```python
from build123d import *

# Parameters (mm, degrees)
F0_W     = 63.5
F0_H     = 5
F1_DEPTH = 10.5
F2_W     = 63.5
F2_H     = 25
F2_H_2   = 5
F3_DEPTH = 5
F4_SIZE  = 4.99999
F5_W     = 63.5
F5_H     = 5
F5_H_2   = 25
F6_DEPTH = 5
F7_SIZE  = 4.99999


# Not quite as in the source:
# - a fillet or chamfer is up to 0.001 mm smaller than in the source, because OpenCascade refuses the exact size


with BuildPart() as f1:
    # F0 (on Top) → F1 (new body)
    with BuildSketch(Plane.XY):
        Rectangle(F0_W, F0_H)
    extrude(amount=F1_DEPTH)

    # F2 (on face) → F3 (join)
    with BuildSketch(Plane.XY.offset(10.5)):
        with Locations((0, -15)):
            Rectangle(F2_W, F2_H)
        Rectangle(F2_W, F2_H_2)
    extrude(amount=F3_DEPTH)

    # F4 (size 5 in the source; OpenCascade refuses exactly that, so slightly less here)
    f4_edges = [f1.edges().sort_by_distance(p)[0] for p in [
        (0, -27.5, 15.5),
    ]]
    chamfer(f4_edges, length=F4_SIZE)

    # F5 (on face) → F6 (join)
    with BuildSketch(Plane(origin=(0, 0, 0), x_dir=(1, 0, 0), z_dir=(0, 0, -1))):
        Rectangle(F5_W, F5_H)
        with Locations((0, 15)):
            Rectangle(F5_W, F5_H_2)
    extrude(amount=F6_DEPTH)

    # F7 (size 5 in the source; OpenCascade refuses exactly that, so slightly less here)
    f7_edges = [f1.edges().sort_by_distance(p)[0] for p in [
        (0, -27.5, -5),
    ]]
    chamfer(f7_edges, length=F7_SIZE)


solid = f1.part
```
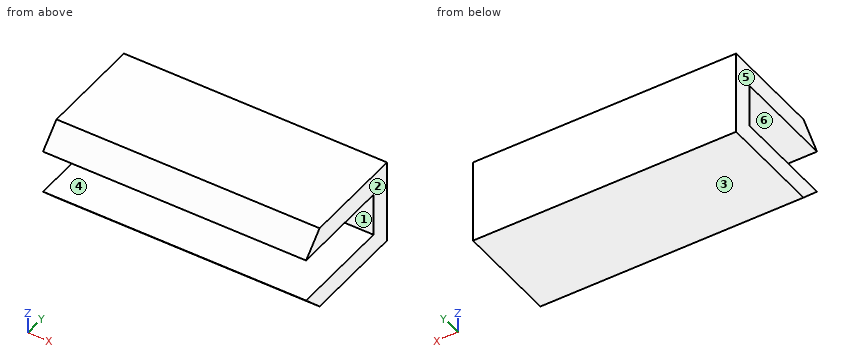
Design review of the part built by this model. Coordinates are the model's own, in mm. Face numbers are marked on the shaded views. A direction names the side the tool comes from. Coordinates: 2 decimals unless noted, no trailing zeros. Order: outer loops, then holes, each group sorted by start corner. A loop starts at its lowest first (then second) coordinate and runs counter-clockwise, first axis right, second up. Notation, with made-up numbers: (72, 75.25) -> (99, 75.25) arc R21 cw to (99, 95.25) -> close; hole circle Ø11 at (-11.5, -34.5). An arc over 180 degrees is marked (long way). One line per item, written item: value. Start each with the question number.
Q1. Tool access review of the marked faces 1 and 2: name each direction out of +Z, -Z, +X, -X, +Y, -Y from which nothing blocks a thin tool from reaching the whole face with its end or side.
Q2. Mouldability with a two-part tool opening along Z and no side actions: class the marked faces 3, 4, 5 and 6 as pulls with the +Z half, pulls with the -Z half, needs draft (parallel to the pull), parting line crosses it, or undercut.
Q3. For probe 1 along Z at (x, y) = (-19.5, -18.5); probe 2 along Y at (x, z) = (23, 9.5); probe 3 along Z at (x, y) = (3, -24.5), list the stretches that pass through material, from the lowest coordinate up.
Q4. Take a section at D-D, the plane z = -1.5. State the section outline as (x, y) points, then the cut area to 3 significant figures.
Q5. Take a section at C-C, the plane z = 6.5. State the section outline as (x, y) points, then the cut area to 4 significant figures.
Q6. Take a section at A-A, the plane y = -14.5. State the section outline as (x, z) points.
Q7. Insertion check: pin 1 Ø8 at (x, z) = (21.5, 4.5) entering from -Y; pin 2 Ø1.5 at (x, z) = (-15.5, -2) entering from -Y; pin 3 Ø12 at (y, z) = (-19.5, 6) entering from -X. Each pin has a flat end and moves straight along its axis. Give the tip position at first contact, or say it passes through.
Values follow:
1. face 1: +X, -X, -Y
1. face 2: +Z, -Z, +X, +Y, -Y
2. face 3: pulls with the -Z half
2. face 4: undercut
2. face 5: needs draft
2. face 6: undercut
3. probe 1: z = -5 to 0, 10.5 to 15.5
3. probe 2: y = -2.5 to 2.5
3. probe 3: z = -3 to 0, 10.5 to 13.5
4. outline: (-31.75, -26) -> (31.75, -26) -> (31.75, 2.5) -> (-31.75, 2.5) -> close
4. area: 1,810 mm2
5. outline: (-31.75, -2.5) -> (31.75, -2.5) -> (31.75, 2.5) -> (-31.75, 2.5) -> close
5. area: 317.5 mm2
6. outline: (-31.75, -5) -> (31.75, -5) -> (31.75, 0) -> (-31.75, 0) -> close; (-31.75, 10.5) -> (31.75, 10.5) -> (31.75, 15.5) -> (-31.75, 15.5) -> close
7. pin 1: stops at y = -2.5
7. pin 2: stops at y = -26.25
7. pin 3: stops at x = -31.75
